```python
from build123d import *

# Parameters (mm, degrees)
F1_DEPTH = 2
F2_W     = 20
F2_H     = 2
F2_W_2   = 2
F2_H_2   = 41
F3_DEPTH = 6
F4_W     = 2
F4_H     = 41
F5_DEPTH = 2


with BuildPart() as f1:
    # F0 (on Top) → F1 (new body)
    with BuildSketch(Plane.XY):
        Polygon((-15, 25), (-25, 25), (-25, -16), (5, -16), (5, -25), (25, -25), (25, -10), (-15, -10), align=None)
    extrude(amount=F1_DEPTH)

    # F2 (on face) → F3 (join)
    with BuildSketch(Plane.XY.offset(2)):
        with Locations((15, -24)):
            Rectangle(F2_W, F2_H)
        with Locations((-24, 4.5)):
            Rectangle(F2_W_2, F2_H_2)
    extrude(amount=F3_DEPTH)

    # F4 (on face) → F5 (join)
    with BuildSketch(Plane.XY.offset(8)):
        with Locations((-24, 4.5)):
            Rectangle(F4_W, F4_H)
        with BuildLine():
            Line((25, 25), (-23, 25))
            Line((-23, 25), (-23, -16))
            Line((-23, -16), (5, -16))
            Line((5, -16), (5, -25))
            Line((5, -25), (25, -25))
            Line((25, -25), (25, -3.5))
            Line((25, -3.5), (-7.4098300563, -3.5))
            ThreePointArc((-7.4098300563, -3.5), (-20.5, 1.5), (-7.4098300563, 6.5))
            Line((-7.4098300563, 6.5), (25, 6.5))
            Line((25, 6.5), (25, 25))
        make_face()
    extrude(amount=F5_DEPTH)


solid = f1.part
```
CAD build for the part. Positions are in the model's coordinates, mm. A direction names the side the tool comes from. Give positions to 0.01 mm unless a question says otherwise; leave off trailing zeros. Order: outer loops, then holes, each group sorted by start corner. A loop starts at its lowest first (then second) coordinate and runs counter-clockwise, first axis right, second up.
(1) Saw through at D-D, the plane x = 7. Give the cut face in (y, z), then the cut area to 3 significant figures.
(2) Flat gauge pins, fed straight in: pin 1 (3 mm diameter, centred on x = 17.5, z = 6, fed in from +Y); pin 2 (2 mm diameter, centred on x = -12, y = 14.5, fed in from -Z); pin 3 (3 mm diameter, centred on y = -4.5, z = 6, fed in from +X). Where does each tip first touch, or does it go through?
(3) Drill centre lines: L1, parallel to Y at x = -13, z = 9.2; L2, parallel to Z at x = -5, y = -13.5; L3, parallel to Y at x = -7, z = 9.25. Where is each one in solid material? Low to high.
(4) Saw through at C-C, the plane z = 1.25. Give the cut face in (x, y).
(5) Tool access for faces 1 (the flat face through (-10.2, -16, 1.6)), 2 (the flat face through (-23, 4, 5)), 3 (the flat face through (1, 7, 8)), 4 (the flat face through (5, -10, 1)): list every direction of +Z, -Z, +X, -X, +Y, -Y with a clear straight run to the whole face (end or side of a thin tool).
(6) Saw through at B-B, the plane y = -20. Give the cut face in (x, z).
(7) Mould opens along Y. For faces 5 (the flat face through (9, 6.5, 9)), 6 (the flat face through (0, 11, 10)), 7 (the flat face through (9, -3.5, 9)), 8 (the flat face through (15, -23, 5)) say: released by +Y, released by -Y, zero draft, split by the parting line, or undercut.
(8) Saw through at A-A, the plane x = -2.5. Give the cut face in (y, z), then the cut area to 3 significant figures.
Results found:
1. outline: (-25, 0) - (-10, 0) - (-10, 2) - (-23, 2) - (-23, 8) - (-3.5, 8) - (-3.5, 10) - (-25, 10) - close; (6.5, 8) - (25, 8) - (25, 10) - (6.5, 10) - close
1. area: 122 mm2
2. pin 1: stops at y = -23
2. pin 2: stops at z = 8
2. pin 3: stops at x = -23
3. L1: y = -16 to -6, 9 to 25
3. L2: z = 0 to 2, 8 to 10
3. L3: y = -16 to -3.5, 6.5 to 25
4. outline: (-25, -16) - (5, -16) - (5, -25) - (25, -25) - (25, -10) - (-15, -10) - (-15, 25) - (-25, 25) - close
5. face 1: +Z, -Z, -X, -Y
5. face 2: +X, +Y, -Y
5. face 3: +X, +Y
5. face 4: -Z, +X, +Y
6. outline: (5, 0) - (25, 0) - (25, 2) - (5, 2) - close; (5, 8) - (25, 8) - (25, 10) - (5, 10) - close
7. face 5: undercut
7. face 6: zero draft
7. face 7: undercut
7. face 8: released by +Y
8. outline: (-16, 0) - (-10, 0) - (-10, 2) - (-16, 2) - close; (-16, 8) - (-3.5, 8) - (-3.5, 10) - (-16, 10) - close; (6.5, 8) - (25, 8) - (25, 10) - (6.5, 10) - close
8. area: 74.0 mm2
